Build history of the part. All positions in model axes, mm. Give positions to 0.01 mm unless a question says otherwise; leave off trailing zeros. Order: outer loops, then holes, each group sorted by start corner. A loop starts at its lowest first (then second) coordinate and runs counter-clockwise, first axis right, second up. Notation, with made-up numbers: (79, 2) -> (133, 2) arc R17 cw to (133, 10) -> close; hole circle Ø9 at (-6, 1.25). An arc over 180 degrees is marked (long way). One line per item, written item: value. Start each with the question number.
(1) Saw through at C-C on z = 1.7. Give the cut face in (x, y), plus the area to 3 significant figures.
(2) Saw through at B-B on x = -137. Give the cut face in (y, z).
(3) Probe line 1 (Y direction, x = -112.5, z = 0.5); line 2 (X direction, y = 60, z = 2.2); line 3 (Y direction, x = -149, z = 0.75). List the from-to ranges inside material, lowest first.
(4) Saw through at A-A on y = -91. Give the cut face in (x, z).
```python
from build123d import *

# Parameters (mm, degrees)
SKETCH1_W          = 357
SKETCH1_H          = 270
SKETCH1_W_2        = 307
SKETCH1_H_2        = 220
EXTRUDE1_DEPTH     = 5
SKETCH3_W          = 6
SKETCH3_H          = 10
CUT_EXTRUDE1_DEPTH = 224.857655665


with BuildPart() as part:
    # Sketch1 → Extrude1 (new body)
    with BuildSketch(Plane.XY):
        Rectangle(SKETCH1_W, SKETCH1_H)
        Rectangle(SKETCH1_W_2, SKETCH1_H_2, mode=Mode.SUBTRACT)
    extrude(amount=EXTRUDE1_DEPTH)

    # Sketch3 → Cut-Extrude1 (cut, through all)
    with BuildSketch(Plane.XY.offset(5)):
        with Locations((-150.5, 115)):
            Rectangle(SKETCH3_W, SKETCH3_H)
        with Locations((150.5, 115)):
            Rectangle(SKETCH3_W, SKETCH3_H)
        with Locations((150.5, -115)):
            Rectangle(SKETCH3_W, SKETCH3_H)
        with Locations((-150.5, -115)):
            Rectangle(SKETCH3_W, SKETCH3_H)
    extrude(amount=-CUT_EXTRUDE1_DEPTH, mode=Mode.SUBTRACT)


solid = part.part
```
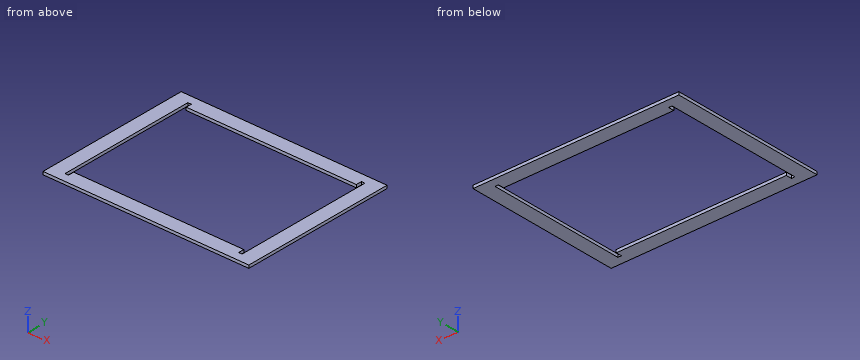
Results below:
1. outline: (-178.5, -135) -> (178.5, -135) -> (178.5, 135) -> (-178.5, 135) -> close; hole (-153.5, -120) -> (-147.5, -120) -> (-147.5, -110) -> (147.5, -110) -> (147.5, -120) -> (153.5, -120) -> (153.5, 120) -> (147.5, 120) -> (147.5, 110) -> (-147.5, 110) -> (-147.5, 120) -> (-153.5, 120) -> close
1. area: 28,600 mm²
2. outline: (-135, 0) -> (-110, 0) -> (-110, 5) -> (-135, 5) -> close; (110, 0) -> (135, 0) -> (135, 5) -> (110, 5) -> close
3. line 1: y = -135 to -110, 110 to 135
3. line 2: x = -178.5 to -153.5, 153.5 to 178.5
3. line 3: y = -135 to -120, 120 to 135
4. outline: (-178.5, 0) -> (-153.5, 0) -> (-153.5, 5) -> (-178.5, 5) -> close; (153.5, 0) -> (178.5, 0) -> (178.5, 5) -> (153.5, 5) -> close
